The model under review builds one solid part; all positions refer to its coordinate system, in mm. A direction names the side the tool comes from. Round coordinates to 2 decimals unless told otherwise and drop trailing zeros. Loops run counter-clockwise (first coordinate to the right, second up) from the corner with the lowest first, then second, coordinate; pieces in that order, holes last. Notation, with made-up numbers: M 66,-29.5 L 103,-29.5 A9 cw 103,-22.5 Z; hole C 8,-15 d1. An arc over 180 degrees is marked long. Return JSON: item names as keys, results as strings. Group by question number.
Q1. To check wall thickness, follow line 1 along Y through (x, z) = (0, -4.25); line 2 along Y through (x, z) = (1.5, 0.25); line 3 along X through (y, z) = (-1, -4.25). State the ranges of each line that lie inside material, in increasing order.
Q2. For faces 3 (the face through (0, -20, 0.5)), 4 (the face through (8.242, -12.623, -3.916)), list the 3-axis set-ups (+Z, -Z, +X, -X, +Y, -Y) from which the entire face can be reached by the end or side of a thin tool; tool diameter is ignored.
Q3. Clearance check with flat-ended pins moving along their axes: pin 1 Ø5.5 at (x, y) = (0, 22.5) entering from +Z; pin 2 Ø3 at (x, y) = (1, -20.5) entering from +Z; pin 3 Ø1.5 at (x, z) = (0.5, -5) entering from +Y. State where each tip first meets the part, or that it passes through.
Q4. Consider section C-C (x = 0.5). State the section outline as (y, z) points, and give its area (3 significant figures).
Q5. Consider section D-D (y = 20). State the section outline as (x, z) points.
Q6. Consider section B-B (y = 8). State the section outline as (x, z) points.
Q7. Draft analysis for pull direction X (two halves, no side actions). For faces 1 (the face through (14.117, -6.017, -4.084)), 2 (the face through (-7, 13, -4)), state which applies: pulls with the +X half, pulls with the -X half, needs draft (parallel to the pull), parting line crosses it, or undercut.
Q8. Consider section A-A (x = -13). State the section outline as (y, z) points.
from build123d import *

# Parameters (mm, degrees)
SKETCH_1_R          = 23.5
EXTRUDE_1_DEPTH     = 2
SKETCH_2_R          = 22.5
EXTRUDE_2_DEPTH     = 10
SKETCH_3_R          = 2
CUT_EXTRUDE_1_DEPTH = 14
SKETCH_5_R          = 5
CUT_EXTRUDE_2_DEPTH = 14
CUT_EXTRUDE_3_DEPTH = 14
FILLET_1_R          = 2
SKETCH_7_R          = 3.5
CUT_EXTRUDE_4_DEPTH = 1.5
SKETCH_8_R          = 11.5
CUT_EXTRUDE_5_DEPTH = 4


with BuildPart() as part:
    # 草图1 → 凸台-拉伸1 (new body)
    with BuildSketch(Plane.XY):
        Circle(SKETCH_1_R)
    extrude(amount=EXTRUDE_1_DEPTH)

    # 草图2 → 凸台-拉伸2 (add)
    with BuildSketch(Plane(origin=(0, 0, 0), x_dir=(-1, 0, 0), z_dir=(0, 0, -1))):
        Circle(SKETCH_2_R)
    extrude(amount=EXTRUDE_2_DEPTH)

    # 草图3 → 切除-拉伸1 (cut)
    with BuildSketch(Plane(origin=(0, 0, -10), x_dir=(-1, 0, 0), z_dir=(0, 0, -1))):
        with Locations((0, 16)):
            Circle(SKETCH_3_R)
        with Locations((13.856406461, -8)):
            Circle(SKETCH_3_R)
        with Locations((-13.856406461, -8)):
            Circle(SKETCH_3_R)
    extrude(amount=-CUT_EXTRUDE_1_DEPTH, mode=Mode.SUBTRACT)

    # 草图5 → 切除-拉伸2 (cut)
    with BuildSketch(Plane(origin=(0, 0, -10), x_dir=(-1, 0, 0), z_dir=(0, 0, -1))):
        Circle(SKETCH_5_R)
    extrude(amount=-CUT_EXTRUDE_2_DEPTH, mode=Mode.SUBTRACT)

    # 草图6 → 切除-拉伸3 (cut)
    with BuildSketch(Plane(origin=(0, 0, -10), x_dir=(-1, 0, 0), z_dir=(0, 0, -1))):
        with BuildLine():
            Line((8.241056104, 17.673001847), (6.127964795, 13.141462912))
            ThreePointArc((6.127964795, 13.141462912), (12.229175964, 7.790844321), (14.5, 0))
            ThreePointArc((14.5, 0), (14.486199213, -0.632481117), (14.444823122, -1.26375827))
            Line((14.444823122, -1.26375827), (19.425796613, -1.699536984))
            ThreePointArc((19.425796613, -1.699536984), (19.481440321, -0.850578054), (19.5, 0))
            ThreePointArc((19.5, 0), (16.446133193, 10.477342363), (8.241056104, 17.673001847))
        make_face()
        with BuildLine():
            Line((11.184740509, -15.973464864), (8.316858327, -11.877704642))
            ThreePointArc((8.316858327, -11.877704642), (0, -14.5), (-8.316858327, -11.877704642))
            Line((-8.316858327, -11.877704642), (-11.184740509, -15.973464864))
            ThreePointArc((-11.184740509, -15.973464864), (0, -19.5), (11.184740509, -15.973464864))
        make_face()
        with BuildLine():
            Line((-19.425796613, -1.699536984), (-14.444823122, -1.26375827))
            ThreePointArc((-14.444823122, -1.26375827), (-12.557368355, 7.25), (-6.127964795, 13.141462912))
            Line((-6.127964795, 13.141462912), (-8.241056104, 17.673001847))
            ThreePointArc((-8.241056104, 17.673001847), (-16.887495374, 9.75), (-19.425796613, -1.699536984))
        make_face()
    extrude(amount=-CUT_EXTRUDE_3_DEPTH, mode=Mode.SUBTRACT)

    # 圆角1
    fillet_1_edges = [part.edges().sort_by_distance(p)[0] for p in [
        (8.241056104, 17.673001847, -4),
        (6.127964795, 13.141462912, -4),
        (14.444823122, -1.26375827, -4),
        (19.425796613, -1.699536984, -4),
        (11.184740509, -15.973464864, -4),
        (8.316858327, -11.877704642, -4),
        (-8.316858327, -11.877704642, -4),
        (-11.184740509, -15.973464864, -4),
        (-19.425796613, -1.699536984, -4),
        (-14.444823122, -1.26375827, -4),
        (-6.127964795, 13.141462912, -4),
        (-8.241056104, 17.673001847, -4),
    ]]
    fillet(fillet_1_edges, radius=FILLET_1_R)

    # 草图7 → 切除-拉伸4 (cut)
    with BuildSketch(Plane.XY.offset(2)):
        with Locations((0, 22.5)):
            Circle(SKETCH_7_R)
        with Locations((19.485571585, -11.25)):
            Circle(SKETCH_7_R)
        with Locations((-19.485571585, -11.25)):
            Circle(SKETCH_7_R)
        with Locations((15.804963619, 9.125)):
            Circle(SKETCH_7_R)
        with Locations((0, -18.25)):
            Circle(SKETCH_7_R)
        with Locations((-15.804963619, 9.125)):
            Circle(SKETCH_7_R)
    extrude(amount=-CUT_EXTRUDE_4_DEPTH, mode=Mode.SUBTRACT)

    # 草图8 → 切除-拉伸5 (cut)
    with BuildSketch(Plane.XY.offset(2)):
        Circle(SKETCH_8_R)
    extrude(amount=-CUT_EXTRUDE_5_DEPTH, mode=Mode.SUBTRACT)


solid = part.part
Values:
{
 "1": {"line 1": "y = -22.5 to -19.5, -14.5 to -5, 5 to 14, 18 to 22.5", "line 2": "y = -23.45 to -19.44, -14.42 to -11.4, 11.4 to 14.68, 17.32 to 23.45", "line 3": "x = -22.48 to -18.84, -15.24 to -4.9, 4.9 to 15.24, 18.84 to 22.48"},
 "2": {"face 3": "+Z", "face 4": "+Z, -Z"},
 "3": {"pin 1": "stops at z = 0.5", "pin 2": "stops at z = 2", "pin 3": "stops at y = 22.5"},
 "4": {"outline": "M -23.49,0 L -22.49,0 L -22.49,-10 L -19.49,-10 L -19.49,0.5 L -21.71,0.5 L -21.71,2 L -23.49,2 Z; M -14.49,-10 L -4.97,-10 L -4.97,-2 L -11.49,-2 L -11.49,2 L -14.49,2 Z; M 4.97,-10 L 14.06,-10 L 14.06,2 L 11.49,2 L 11.49,-2 L 4.97,-2 Z; M 17.94,-10 L 22.49,-10 L 22.49,0 L 23.49,0 L 23.49,0.5 L 19.04,0.5 L 19.04,2 L 17.94,2 Z", "area": "256 mm2"},
 "5": {"outline": "M -12.34,0 L -10.31,0 L -10.31,-10 L 10.31,-10 L 10.31,0 L 12.34,0 L 12.34,2 L 2.45,2 L 2.45,0.5 L -2.45,0.5 L -2.45,2 L -12.34,2 Z"},
 "6": {"outline": "M -22.1,0 L -21.03,0 L -21.03,-10 L -17.78,-10 L -17.78,0.5 L -19.12,0.5 L -19.12,2 L -22.1,2 Z; M -12.09,-10 L 12.09,-10 L 12.09,2 L 8.26,2 L 8.26,-2 L -8.26,-2 L -8.26,2 L -12.09,2 Z; M 17.78,-10 L 21.03,-10 L 21.03,0 L 22.1,0 L 22.1,2 L 19.12,2 L 19.12,0.5 L 17.78,0.5 Z"},
 "7": {"face 1": "undercut", "face 2": "undercut"},
 "8": {"outline": "M -19.58,0 L -18.36,0 L -18.36,-10 L -9.81,-10 L -9.81,2 L -19.58,2 Z; M -6.19,-10 L 6.42,-10 L 6.42,2 L -6.19,2 Z; M 14.53,-10 L 18.36,-10 L 18.36,0 L 19.58,0 L 19.58,2 L 14.53,2 Z"}
}
